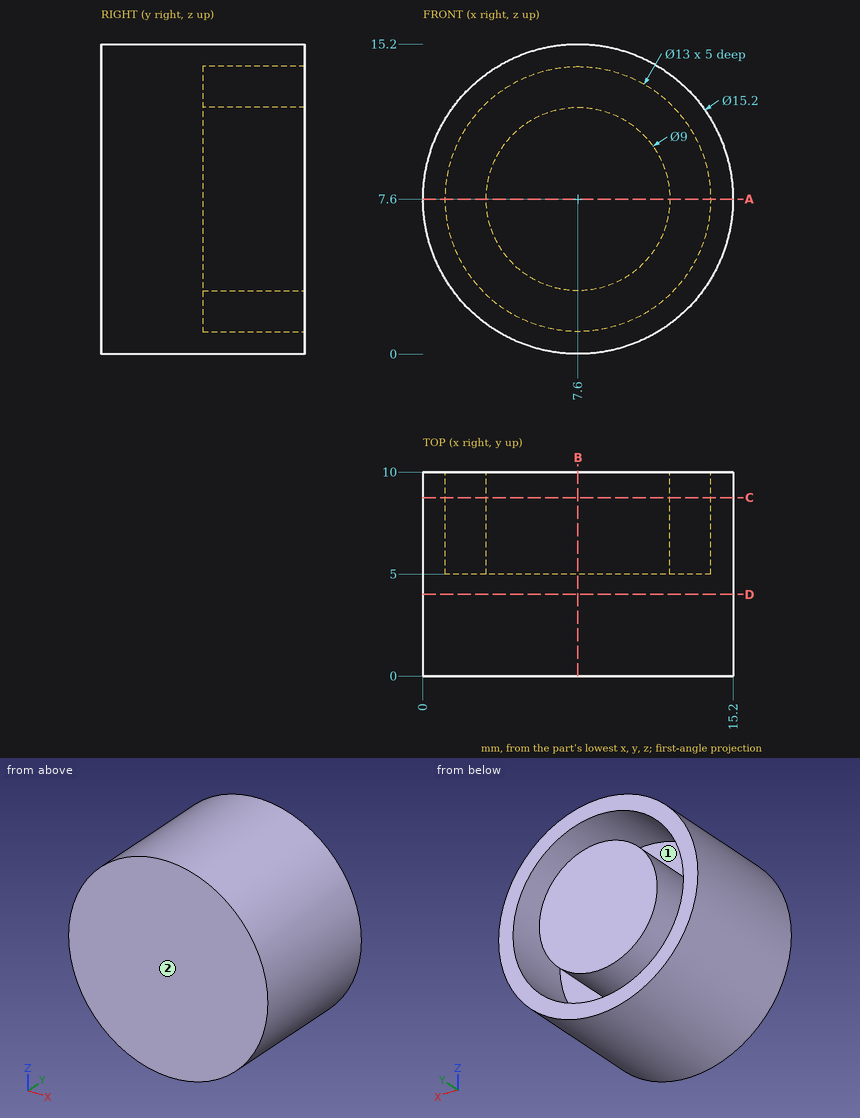
Study the drawing (mm; zero at the part's minimum x, y, z) and answer. A direction names the side the tool comes from. Coordinates: 2 decimals unless noted, no trailing zeros. Loops run counter-clockwise (first coordinate to the right, second up) from the corner with the lowest first, then second, coordinate; pieces in that order, holes last. Notation, with made-up numbers: M -28,63 L -21,63 A20 ccw -21,97 Z; hole C 56,-3 d8. An arc over 180 degrees is marked long. Answer in a Markdown table with one row per item. Add a question column.
1. Consider L1, parallel to X at y = 8.6, z = 7.6; L2, parallel to Z at x = 6, y = 8; L3, parallel to Z at x = 11, y = 7.5. Determine where each line is inside the solid, lowest interval first.
2. Flat-ended cylindrical pins translate along their axes: P1, Ø4, axis at x = 13, y = 6, coming from the -Z side; P2, Ø6, axis at y = 9, z = 3.5, coming from the -X side; P3, Ø1, axis at y = 3.5, z = 13.5, coming from the +X side. Find the tip coordinate at first contact, or state that the pin passes through.
3. Find section C-C, the plane y = 8.75. Write down the section's boundary in (x, z).
4. Find section D-D, the plane y = 4. Write down the section's boundary in (x, z).
5. Find section A-A, the plane z = 7.6. Write down the section's boundary in (x, y), then the cut area to 3 significant figures.
6. A tool of negligible diameter and unlimited length cuts with its end or side. For the marked faces 1 and 2, from which of +Z, -Z, +X, -X, +Y, -Y can it reach the whole face along a straight path? Write none if from no direction.
7. Find section B-B, the plane x = 7.6. Write down the section's boundary in (y, z), then the cut area to 3 significant figures.
Reported:
| question | item | result |
|---|---|---|
| 1 | L1 | x = 0 to 1.1, 3.1 to 12.1, 14.1 to 15.2 |
| 1 | L2 | z = 0.17 to 1.3, 3.39 to 11.81, 13.9 to 15.03 |
| 1 | L3 | z = 0.8 to 2.06, 4.65 to 10.55, 13.14 to 14.4 |
| 2 | P1 | stops at z = 0.8 |
| 2 | P2 | stops at x = 0.08 |
| 2 | P3 | stops at x = 12.95 |
| 3 | outline | C 7.6,7.6 d15.2; C 7.6,7.6 d9; hole C 7.6,7.6 d13 |
| 4 | outline | C 7.6,7.6 d15.2 |
| 5 | outline | M 0,0 L 15.2,0 L 15.2,10 L 14.1,10 L 14.1,5 L 12.1,5 L 12.1,10 L 3.1,10 L 3.1,5 L 1.1,5 L 1.1,10 L 0,10 Z |
| 5 | area | 132 mm^2 |
| 6 | face 1 | +Y |
| 6 | face 2 | +Z, -Z, +X, -X, -Y |
| 7 | outline | M 0,0 L 10,0 L 10,1.1 L 5,1.1 L 5,3.1 L 10,3.1 L 10,12.1 L 5,12.1 L 5,14.1 L 10,14.1 L 10,15.2 L 0,15.2 Z |
| 7 | area | 132 mm^2 |
